Drawing for the job (mm, zero at the part's lowest x, y, z). A direction names the side the tool comes from. Give positions to 0.01 mm unless a question says otherwise; leave off trailing zeros. Order: outer loops, then holes, each group sorted by start corner. A loop starts at its lowest first (then second) coordinate and runs counter-clockwise, first axis right, second up. Notation, with made-up numbers: M 6,42 L 16,42 A20 cw 16,69 Z; hole C 12,4.5 d6. An arc over 180 degrees is marked long. One line per item, written item: value.
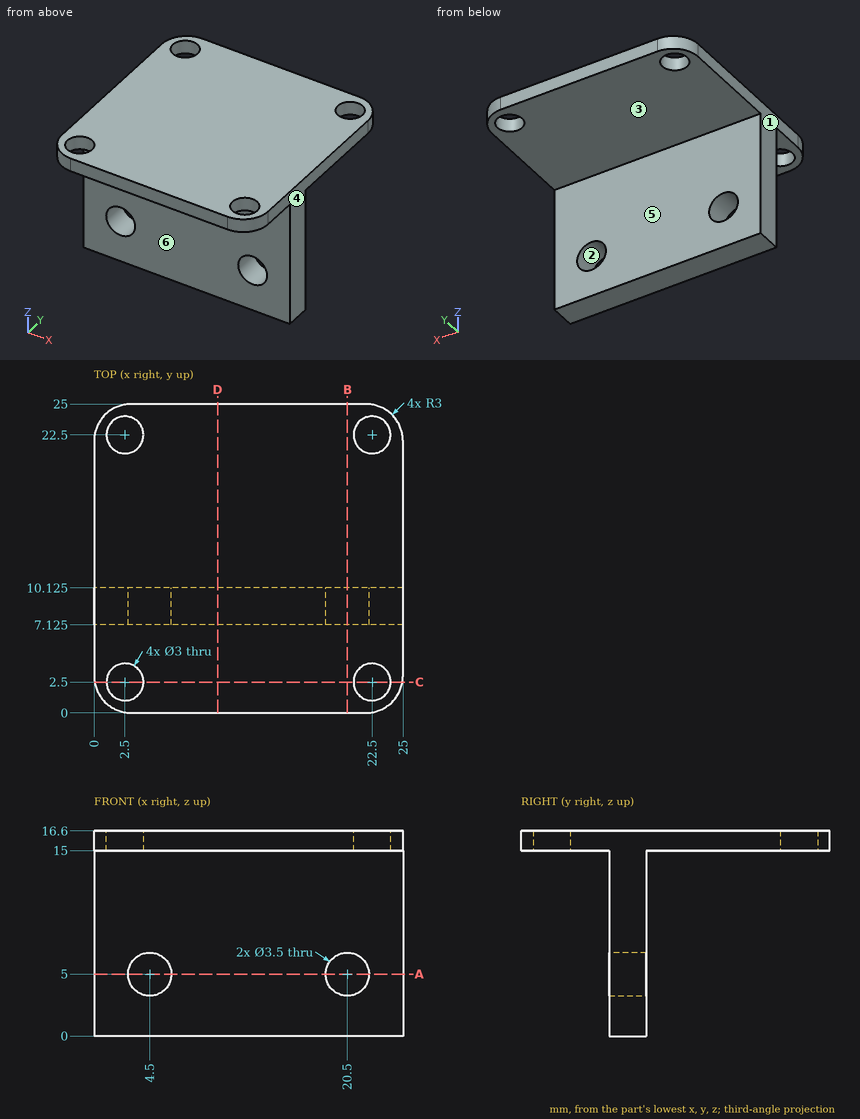
1) Pin check, flat tips, straight feed: pin 1 (4.5 mm diameter, centred on x = 11.5, z = 9, fed in from +Y) (3 decimals); pin 2 (3 mm diameter, centred on x = 4.5, z = 5, fed in from -Y); pin 3 (8 mm diameter, centred on x = 8.5, z = 2, fed in from -Y) (3 decimals); pin 4 (1 mm diameter, centred on x = 17, y = 4.5, fed in from -Z). Stop position of each tip, or through.
Check values:
pin 1: y = 10.125
pin 2: through
pin 3: y = 7.125
pin 4: z = 15
2) Saw through at D-D, the plane x = 10. Write the cut outline in (y, z) (3 decimals).
Check values:
outline: M 0,15 L 7.125,15 L 7.125,0 L 10.125,0 L 10.125,15 L 25,15 L 25,16.6 L 0,16.6 Z
3) Saw through at B-B, the plane x = 20.5. Write the cut outline in (y, z) (3 decimals).
Check values:
outline: M 0,15 L 7.125,15 L 7.125,6.75 L 10.125,6.75 L 10.125,15 L 25,15 L 25,16.6 L 0,16.6 Z; M 7.125,0 L 10.125,0 L 10.125,3.25 L 7.125,3.25 Z
4) Saw through at A-A, the plane z = 5. Write the cut outline in (x, y) (3 decimals).
Check values:
outline: M 0,7.125 L 2.75,7.125 L 2.75,10.125 L 0,10.125 Z; M 6.25,7.125 L 18.75,7.125 L 18.75,10.125 L 6.25,10.125 Z; M 22.25,7.125 L 25,7.125 L 25,10.125 L 22.25,10.125 Z
5) Mould opens along Z. For the marked faces 1, 2 and 3 say: released by +Z, released by -Z, zero draft, split by the parting line, or undercut.
Check values:
face 1: zero draft
face 2: undercut
face 3: released by -Z
6) Tool access for the marked faces 4, 5 and 6: list every direction of +Z, -Z, +X, -X, +Y, -Y with a clear straight run to the whole face (end or side of a thin tool).
Check values:
face 4: +Z, -Z, +X, +Y, -Y
face 5: -Z, +X, -X, +Y
face 6: -Z, +X, -X, -Y
7) Drill centre lines: probe 1 along X at (y, z) = (8.4, 5); probe 2 along Y at (x, z) = (22.5, 15.4); probe 3 along Z at (x, y) = (16.75, 3). Where is each one in solid material? Low to high. Write a range as from..to.
Check values:
probe 1: 0..2.75, 6.25..18.75, 22.25..25
probe 2: 0.04..1, 4..21, 24..24.96
probe 3: 15..16.6
8) Saw through at C-C, the plane y = 2.5. Write the cut outline in (x, z).
Check values:
outline: M 0.04,15 L 1,15 L 1,16.6 L 0.04,16.6 Z; M 4,15 L 21,15 L 21,16.6 L 4,16.6 Z; M 24,15 L 24.96,15 L 24.96,16.6 L 24,16.6 Z
